from build123d import *

# Parameters (mm, degrees)
SKETCH1_R           = 1.5875
BOSS_EXTRUDE1_DEPTH = 1.5875


with BuildPart() as part:
    # Sketch1 → Boss-Extrude1 (new body, symmetric)
    with BuildSketch(Plane.XY):
        with BuildLine():
            Line((-5.08, 0), (-5.08, -5.737908239))
            ThreePointArc((-5.08, -5.737908239), (-4.973712071, -6.309018604), (-4.669080882, -6.803653836))
            Line((-4.669080882, -6.803653836), (-1.111541176, -10.731170137))
            ThreePointArc((-1.111541176, -10.731170137), (2.803287219, -11.66181504), (5.08, -8.3439))
            Line((5.08, -8.3439), (5.08, 0))
            Line((5.08, 0), (2.38125, 0))
            Line((2.38125, 0), (2.38125, 3.175))
            Line((2.38125, 3.175), (-2.38125, 3.175))
            Line((-2.38125, 3.175), (-2.38125, 0))
            Line((-2.38125, 0), (-5.08, 0))
        make_face()
        with Locations((1.524, -8.3439)):
            Circle(SKETCH1_R, mode=Mode.SUBTRACT)
    extrude(amount=BOSS_EXTRUDE1_DEPTH, both=True)


solid = part.part
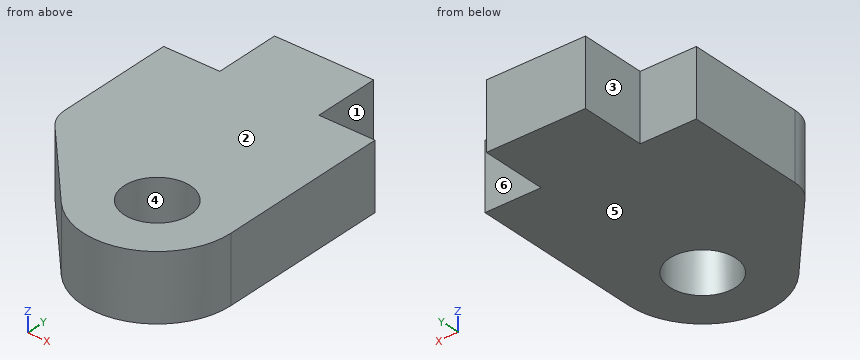
Input: part model. Units: mm. Frame: model coordinates. Face numbers are marked on the shaded views. A direction names the side the tool comes from. Give positions to 0.01 mm unless a question says otherwise; leave off trailing zeros. Order: outer loops, then holes, each group sorted by start corner. A loop starts at its lowest first (then second) coordinate and runs counter-clockwise, first axis right, second up.
Q1. Set-up query: the marked faces 1, 2 and 3. Return all of +Z, -Z, +X, -X, +Y, -Y with unobstructed straight access to the full face (end or side cutting, diameter ignored); none if empty.
Checked values:
face 1: +Z, -Z, +X, +Y
face 2: +Z, +X, -X, +Y, -Y
face 3: +Z, -Z, -X, +Y
Q2. Section D-D on x = -3.75. Output: boundary loops of the cut face in (y, z).
Checked values:
outline: (-7.82, -1.59) - (0, -1.59) - (0, 1.59) - (-7.82, 1.59) - close
Q3. Draft query along Y for the marked faces 4, 5 and 6. Return one class per face: +Y half, -Y half, draft (parallel to the pull), parting line (faces both ways), or undercut.
Checked values:
face 4: undercut
face 5: draft
face 6: +Y half
Q4. Contact query for flat-ended pins moving along their axis: pin 1 Ø1 at (x, z) = (-2.5, 0) entering from +Y (3 decimals); pin 2 Ø1.9 at (x, y) = (1.52, -8.34) entering from -Z; pin 3 Ø1.6 at (y, z) = (1.5, 0.5) entering from -X; pin 4 Ø1 at (y, z) = (2, -0.5) entering from +X. Output: stop coordinate, or through.
Checked values:
pin 1: stops at y = 3.175
pin 2: passes through
pin 3: stops at x = -2.38
pin 4: stops at x = 2.38
Q5. Section B-B on y = -8. Output: boundary loops of the cut face in (x, z).
Checked values:
outline: (-3.59, -1.59) - (-0.03, -1.59) - (-0.03, 1.59) - (-3.59, 1.59) - close; (3.07, -1.59) - (5.08, -1.59) - (5.08, 1.59) - (3.07, 1.59) - close
Q6. Ray query, probe 1 along X at (y, z) = (1.25, 0.7); probe 2 along Y at (x, z) = (2.5, 1.15); probe 3 along Y at (x, z) = (1, -0.95) (3 decimals). Return the intervals inside material, ascending.
Checked values:
probe 1: x = -2.38 to 2.38
probe 2: y = -11.76 to -9.6, -7.09 to 0
probe 3: y = -11.861 to -9.842, -6.845 to 3.175
Q7. Section C-C on z = -1. Output: boundary loops of the cut face in (x, y) (1 decimal), and give its area (3 significant figures).
Checked values:
outline: (-5.1, -5.7) arc R1.6 ccw to (-4.7, -6.8) - (-1.1, -10.7) arc R3.6 ccw to (5.1, -8.3) - (5.1, 0) - (2.4, 0) - (2.4, 3.2) - (-2.4, 3.2) - (-2.4, 0) - (-5.1, 0) - close; hole circle Ø3.2 at (1.5, -8.3)
area: 111 mm2
Q8. Section A-A on x = 1.25. Output: boundary loops of the cut face in (y, z) (1 decimal).
Checked values:
outline: (-11.9, -1.6) - (-9.9, -1.6) - (-9.9, 1.6) - (-11.9, 1.6) - close; (-6.8, -1.6) - (3.2, -1.6) - (3.2, 1.6) - (-6.8, 1.6) - close
